The model under review builds one solid part; all positions refer to its coordinate system, in mm. Face numbers are marked on the shaded views. A direction names the side the tool comes from. Round coordinates to 2 decimals unless told otherwise and drop trailing zeros. Loops run counter-clockwise (first coordinate to the right, second up) from the corner with the lowest first, then second, coordinate; pieces in that order, holes last. Notation, with made-up numbers: (77.25, 81) - (114.25, 81) arc R16 cw to (114.25, 105) - close; hole circle Ø11 at (50.25, -30). An arc over 180 degrees is marked (long way). Answer as CSV lines item,"result".
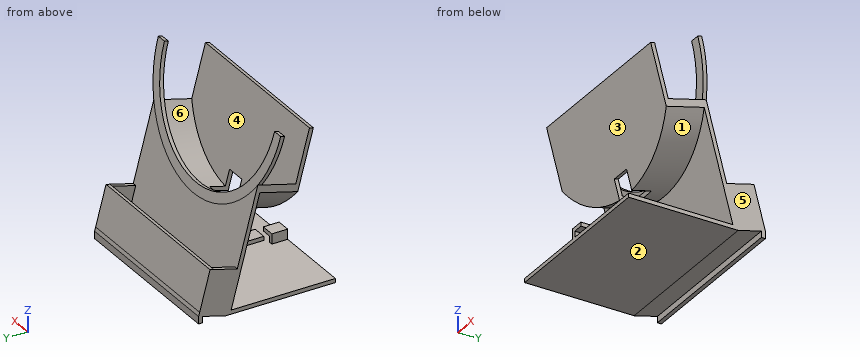
from build123d import *

# Parameters (mm, degrees)
F1_DEPTH  = 85
F3_DEPTH  = 2
F5_DEPTH  = 2
F7_DEPTH  = 25
F9_DEPTH  = 17.5
F11_DEPTH = 2
F13_DEPTH = 10
F15_DEPTH = 2
F16_W     = 7
F16_H     = 10
F17_DEPTH = 5
F18_W     = 5
F18_H     = 3
F19_DEPTH = 25
F20_W     = 7
F20_H     = 7.8445977569
F21_DEPTH = 5
F22_W     = 5
F22_H     = 3
F23_DEPTH = 8


with BuildPart() as f1:
    # F0 (on Right) → F1 (new body)
    with BuildSketch(Plane.YZ):
        Polygon((-54.3862693012, 2), (-54.3862693012, 0), (0, 0), (11.522961568, 3.0875682466), (11.522961568, 0), (13.522961568, 0), (13.522961568, 3.6234666314), (13.0053234778, 5.555318284), (7.8289425758, 24.8738348098), (5.8970909232, 24.3561967196), (11.0734718253, 5.0376801938), (-0.5176380902, 1.9318516526), (-23.2389682748, 86.7290103171), (-25.1708199274, 86.2113722269), (-2.6064507457, 2), align=None)
    extrude(amount=F1_DEPTH)

    # F2 (on face) → F3 (join)
    with BuildSketch(Plane.YZ.offset(85)):
        Polygon((11.0734718253, 5.0376801938), (5.8970909232, 24.3561967196), (-5.6940189923, 21.2503681784), (-0.5176380902, 1.9318516526), align=None)
    extrude(amount=-F3_DEPTH)

    # F4 (on face) → F5 (join)
    with BuildSketch(Plane(origin=(0, 0, 0), x_dir=(0, -1, 0), z_dir=(-1, 0, 0))):
        Polygon((5.6940189923, 21.2503681784), (-5.8970909232, 24.3561967196), (-11.0734718253, 5.0376801938), (0.5176380902, 1.9318516526), align=None)
    extrude(amount=-F5_DEPTH)

    # F6 (on face) → F7 (cut)
    with BuildSketch(Plane(origin=(0, -1.9318516526, -0.5176380902), x_dir=(1, 0, 0), z_dir=(0, -0.9659258263, -0.2588190451))):
        with BuildLine():
            ThreePointArc((0, 61.2673163635), (56.1930639376, 39.5179905915), (92.5, 87.6064507457))
            ThreePointArc((92.5, 87.6064507457), (28.8069360624, 135.6949108999), (0, 61.2673163635))
        make_face()
    extrude(amount=-F7_DEPTH, mode=Mode.SUBTRACT)

    # F8 (on face) → F9 (join)
    with BuildSketch(Plane(origin=(0, -1.9318516526, -0.5176380902), x_dir=(1, 0, 0), z_dir=(0, -0.9659258263, -0.2588190451))):
        with BuildLine():
            ThreePointArc((85, 61.2673163636), (42.5, 37.6064507457), (0, 61.2673163636))
            Line((0, 61.2673163636), (0, 57.6439742125))
            ThreePointArc((0, 57.6439742125), (42.5, 35.6064507457), (85, 57.6439742125))
            Line((85, 57.6439742125), (85, 61.2673163636))
        make_face()
    extrude(amount=F9_DEPTH)

    # F10 (on face) → F11 (join)
    with BuildSketch(Plane(origin=(0, -18.8355536126, -5.0469713795), x_dir=(1, 0, 0), z_dir=(0, -0.9659258263, -0.2588190451))):
        with BuildLine():
            Line((0, 61.2673163636), (0, 57.6439742125))
            ThreePointArc((0, 57.6439742125), (42.5, 35.6064507457), (85, 57.6439742125))
            Line((85, 57.6439742125), (85, 61.2673163636))
            Line((85, 61.2673163636), (85, 87.6064507457))
            Line((85, 87.6064507457), (0, 87.6064507457))
            Line((0, 87.6064507457), (0, 61.2673163636))
        make_face()
    extrude(amount=F11_DEPTH)

    # F12 (on face) → F13 (cut)
    with BuildSketch(Plane(origin=(0, -20.7674052652, -5.5646094697), x_dir=(1, 0, 0), z_dir=(0, -0.9659258263, -0.2588190451))):
        with BuildLine():
            Line((37.5, 45.8473935673), (37.5, 35.8473935673))
            ThreePointArc((37.5, 35.8473935673), (42.5, 35.6064507457), (47.5, 35.8473935673))
            Line((47.5, 35.8473935673), (47.5, 45.8473935673))
            Line((47.5, 45.8473935673), (37.5, 45.8473935673))
        make_face()
    extrude(amount=-F13_DEPTH, mode=Mode.SUBTRACT)

    # F14 (on face) → F15 (join)
    with BuildSketch(Plane(origin=(0, 0, 0), x_dir=(-1, 0, 0), z_dir=(0, 0.9659258263, 0.2588190451))):
        with BuildLine():
            ThreePointArc((-92.5, 87.6064507457), (-42.5, 37.6064507457), (7.5, 87.6064507457))
            Line((7.5, 87.6064507457), (2.5, 87.6064507457))
            ThreePointArc((2.5, 87.6064507457), (-42.5, 42.6064507457), (-87.5, 87.6064507457))
            Line((-87.5, 87.6064507457), (-92.5, 87.6064507457))
        make_face()
    extrude(amount=-F15_DEPTH)

    # F16 (on face) → F17 (join)
    with BuildSketch(Plane.XY.offset(2)):
        with Locations((42.5, -37.5416715443)):
            Rectangle(F16_W, F16_H)
    extrude(amount=F17_DEPTH)

    # F18 (on face) → F19 (cut)
    with BuildSketch(Plane.XZ.offset(42.5416715443)):
        with Locations((41.5, 3.5)):
            Rectangle(F18_W, F18_H)
    extrude(amount=-F19_DEPTH, mode=Mode.SUBTRACT)

    # F20 (on face) → F21 (join)
    with BuildSketch(Plane.XY.offset(2)):
        with Locations((42.5, -50.4639704227)):
            Rectangle(F20_W, F20_H)
    extrude(amount=F21_DEPTH)

    # F22 (on face) → F23 (cut)
    with BuildSketch(Plane.XZ.offset(54.3862693012)):
        with Locations((43.5, 3.5)):
            Rectangle(F22_W, F22_H)
    extrude(amount=-F23_DEPTH, mode=Mode.SUBTRACT)


solid = f1.part
1. Draft analysis for pull direction Y (two halves, no side actions). For the marked faces 3, 4, 5 and 6, state which applies: +Y half, -Y half, draft (parallel to the pull), parting line (faces both ways), or undercut.
Numbers:
face 3,"-Y half"
face 4,"undercut"
face 5,"draft"
face 6,"undercut"
2. Take a section at C-C (y = -8.5). State the section outline as (x, z) points, plus the area to 3 significant figures.
Numbers:
outline,"(0, 0) - (85, 0) - (85, 2) - (0, 2) - close; (0, 24) - (85, 24) - (85, 31.72) - (0, 31.72) - close"
area,"827 mm²"
3. Take a section at D-D (y = -19). State how many separate pieces and enclosed holes the cut face has, plus the area to 3 significant figures.
Numbers:
separate pieces,"4"
enclosed holes,"0"
area,"462 mm²"
4. Take a section at B-B (x = 73). State the section outline as (y, z) points.
Numbers:
outline,"(-54.39, 0) - (0, 0) - (11.52, 3.09) - (11.52, 0) - (13.52, 0) - (13.52, 3.62) - (7.83, 24.87) - (5.9, 24.36) - (11.07, 5.04) - (-0.52, 1.93) - (-14.11, 52.66) - (-16.04, 52.14) - (-14.35, 45.83) - (-31.26, 41.3) - (-41.51, 79.57) - (-43.44, 79.06) - (-32.54, 38.38) - (-13.71, 43.42) - (-2.61, 2) - (-54.39, 2) - close"
5. Clearance check with flat-ended pins moving along their axes: pin 1 (5 mm diameter, centred on y = -28, z = 36, fed in from +X); pin 2 (8 mm diameter, centred on x = 46.5, z = 33.5, fed in from +Y); pin 3 (1.5 mm diameter, centred on y = -35.5, z = 42, fed in from +X); pin 4 (1.5 mm diameter, centred on y = -49, z = 4.5, fed in from -X). State where each tip first meets the part, or that it passes through.
Numbers:
pin 1,"stops at x = 71.61"
pin 2,"stops at y = -7.9"
pin 3,"passes through"
pin 4,"stops at x = 39"
6. Tool access review of the marked faces 1 and 2: name each direction out of +Z, -Z, +X, -X, +Y, -Y from which nothing blocks a thin tool from reaching the whole face with its end or side.
Numbers:
face 1,"none"
face 2,"-Z, +X, -X, +Y, -Y"
7. Take a section at A-A (y = -39). State the section outline as (x, z) points, plus the area to 3 significant figures.
Numbers:
outline,"(0, 0) - (85, 0) - (85, 2) - (46, 2) - (46, 7) - (39, 7) - (39, 5) - (44, 5) - (44, 2) - (0, 2) - close; (0, 62.48) - (85, 62.48) - (85, 70.21) - (0, 70.21) - close"
area,"847 mm²"
8. Wall thickness on probe 1 along Z at (x, y) = (46.5, -45); probe 2 along Y at (x, z) = (18, 11); probe 3 along Z at (x, y) = (49.5, -21): over which ranges is each line inside the solid? List them lowest first.
Numbers:
probe 1,"z = 0 to 2"
probe 2,"y = -5.02 to -2.95, 9.48 to 11.55"
probe 3,"z = 0 to 2, 31.73 to 33.82"
